Can you work these out from the drawing? Everything is in mm from the part's minimum corner. Round coordinates to 2 decimals unless told otherwise and drop trailing zeros. Order: outer loops, then holes, each group sorted by start corner. A loop starts at its lowest first (then second) coordinate and runs counter-clockwise, first axis right, second up. Notation, with made-up numbers: (42.25, 69.25) -> (96.25, 69.25) arc R23 ccw to (96.25, 99.25) -> close; hole circle Ø10 at (71, 80.25). An arc over 180 degrees is marked (long way). One line per item, written item: value.
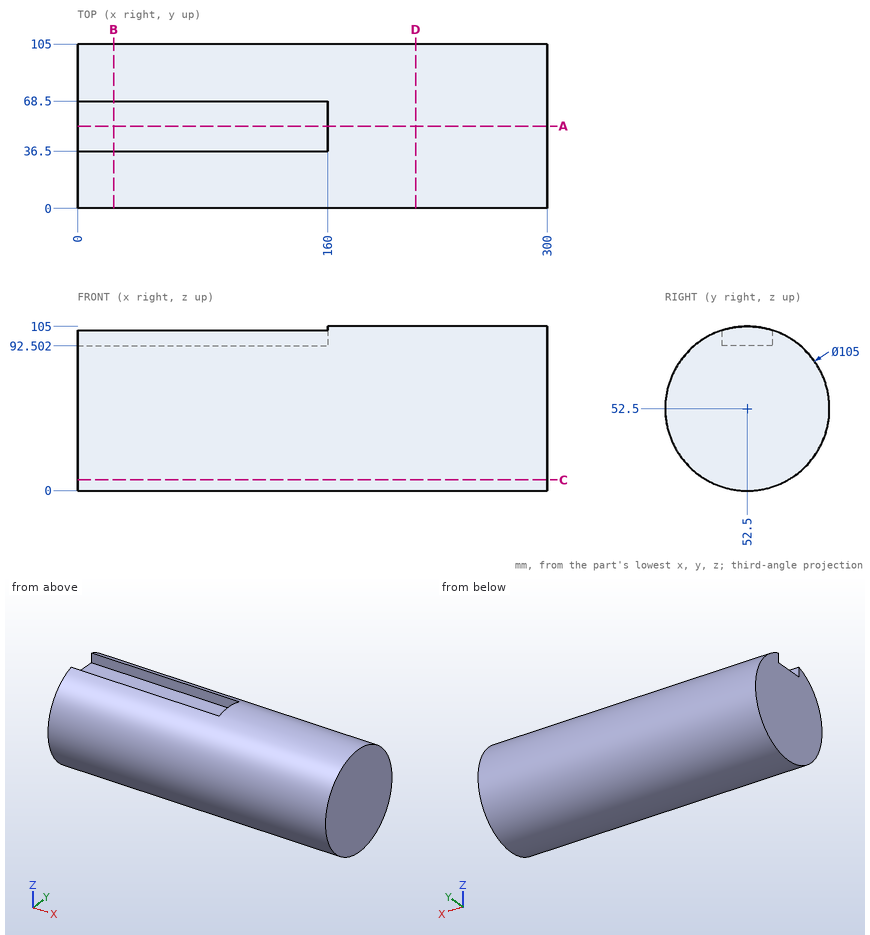
Q1. I want a section at B-B on x = 23. List the corners of the cut face in (y, z) for me.
Answers below:
outline: (36.5, 92.5) -> (36.5, 102.5) arc R52.5 ccw (long way) to (68.5, 102.5) -> (68.5, 92.5) -> close
Q2. I want a section at C-C on z = 7. List the corners of the cut face in (x, y) for me.
Answers below:
outline: (0, 26.31) -> (300, 26.31) -> (300, 78.69) -> (0, 78.69) -> close
Q3. I want a section at D-D on x = 216. List the corners of the cut face in (y, z) for me, plus the area to 3 significant figures.
Answers below:
outline: circle Ø105 at (52.5, 52.5)
area: 8,660 mm^2
Q4. I want a section at A-A on y = 52.5. List the corners of the cut face in (x, z) for me, plus the area to 3 significant figures.
Answers below:
outline: (0, 0) -> (300, 0) -> (300, 105) -> (160, 105) -> (160, 92.5) -> (0, 92.5) -> close
area: 29,500 mm^2
Q5. Please list where these lines run through material, in increasing order: line 1 along Z through (x, y) = (48.5, 52.5); line 2 along Y through (x, z) = (240, 24); line 3 along Z through (x, y) = (69, 79.5) (1 decimal).
Answers below:
line 1: 0 to 92.5
line 2: 8.41 to 96.59
line 3: 7.5 to 97.5
Q6. Will these pins go through, and if not, where does the flat tip stop? pin 1 Ø1.5 at (x, z) = (198.5, 16.5) entering from +Y (1 decimal); pin 2 Ø9.5 at (x, y) = (58.5, 50) entering from +Z; pin 3 Ø8 at (x, z) = (213, 89) entering from +Y.
Answers below:
pin 1: y = 91.4
pin 2: z = 92.5
pin 3: y = 93.73
